Autodesk Inventor part; units mm, degrees
ref_plane "Work Plane1" through (29, 0, 0) normal (0, -1, 0) x (1, 0, 0)
ref_plane "YZ Plane" through (0, 0, 0) normal (1, 0, 0) x (0, 1, 0)
ref_plane "XZ Plane" through (0, 0, 0) normal (0, 1, 0) x (-1, 0, 0)
sketch "Sketch1" plane through (0, 0, 0) normal (0, 0, 1) x (1, 0, 0)
  line L0 (-0.7535, 0) -> (15.875, 0)
  line L1 (15.875, 0) -> (15.875, 1.4224)
  line L2 (15.875, 1.4224) -> (1.5877, 1.4224)
  line L3 (1.5877, 1.4224) -> (0.0001, 1.4224)
  line L4 (0.0001, 1.4224) -> (0, 1.4224)
  line L5 (0, 1.4224) -> (0, 2.3241)
  line L6 (0, 2.3241) -> (-2.8448, 2.3241)
  line L7 (-2.8448, 2.3241) -> (-2.8448, 1.3785)
  line L8 (-2.8448, 1.3785) -> (-1.5494, 1.3785)
  line L9 (-1.5494, 1.3785) -> (-0.7535, 0)
  line L10 (-6.5888, 0) -> (19.619, 0)
  line L11 (0, -0.4648) -> (0, 2.7889)
  line L12 (1.5877, 1.4224) -> (0, 1.4224) construction
  dimension "d1" = 14.2873
  dimension "d2" = 1.5876
  dimension "d3" = 2.8448
  dimension "d4" = 1.2954
  dimension "d5" = 60
  dimension "d6" = 2.8448
  dimension "d7" = 2.8448
  dimension "d8" = 2.757
  dimension "d9" = 4.6482
  dimension "d26" = 15.875
revolve "Body" add sketch "Sketch1" angle 360 about axis through (-0.7535, 0, 0) along (1, 0, 0)
sketch "Sketch2" plane through (-2.8448, 0, 0) normal (-1, 0, 0) x (0, 0, 1)
  circle A0 centre (0, 0) radius 1.3785
  line L0 (0, -3.2537) -> (0, 3.2537)
  line L1 (-3.2537, 0) -> (3.2537, 0)
  line L2 (1.3785, 0) -> (0.6892, -1.1938)
  line L3 (0.6892, -1.1938) -> (-0.6892, -1.1938)
  line L4 (-0.6892, -1.1938) -> (-1.3785, 0)
  line L5 (-1.3785, 0) -> (-0.6892, 1.1938)
  line L6 (-0.6892, 1.1938) -> (0.6892, 1.1938)
  line L7 (0.6892, 1.1938) -> (1.3785, 0)
  point P0 (0, 0)
extrude "Slot" add sketch "Sketch2" against normal up to next contours L7 A0 | A0 L2 | L6 L0 A0 | A0 L0 L3 | L0 L6 A0 | A0 L3 L0 | L4 A0 | A0 L5
fillet "Fillet1" radius 0.2286 1 edges at (-2.8448, -2.3241, 0)
thread "Thread"
chamfer "Chamfer1" distance 0.3785 distance2 0.3785 1 edges at (15.875, -1.4224, 0) measured on face at (15.875, -0.3591, -0.7201)
ref_plane "Work Plane1" through (29, 0, 0) normal (0, -1, 0) x (1, 0, 0)
fillet "Fillet2" radius 0.1016 1 edges at (0.0001, -1.4224, 0)
equation "\"d1\" = GEL"
equation "\"d3\" = KOH"
equation "\"d4\" = INTI"
equation "\"d6\" = GD"
equation "\"d7\" = BDM"
equation "\"d8\" = 1.1547 * SW"
equation "\"d9\" = KOD"
equation "\"d26\" = NLG"
equation "\"d30\" = R"
equation "\"d17\" = RR"
equation "\"d13\" = GEL"
equation "\"d15\" = -0.5 * SPD + 0.5 * GD"
equation "\"d16\" = GUL"
equation "\"GD\" = 2.8448"
equation "\"NLG\" = 15.875"
equation "\"GEL\" = 14.2873"
equation "\"KOD\" = 4.6482"
equation "\"KOH\" = 2.8448"
equation "\"INTI\" = 1.2954"
equation "\"GAL\" = 1.5875"
equation "\"GUL\" = 0.37846"
equation "\"BDM\" = 2.8448"
equation "\"SW\" = 2.3876"
equation "\"RR\" = 0.2286"
equation "\"SPD\" = 2.08788"
equation "\"R\" = 0.1016"
equation "\"PHH\" = 0.127"
equation "\"GD1\" = SPD"
equation "\"THREADDIA\" = 2.8448"
equation "\"FAWI\" = 45deg"
equation "\"KOH1\" = 2.5654"
equation "\"NND\" = 2.8448"
equation "\"TOA\" = 30deg"
equation "\"E0\" = 1.155 * SW"
properties part number "ANSI B18.3 - No. 4 - 40 UNC - 5/8 HS HCS" material "Steel, Mild"
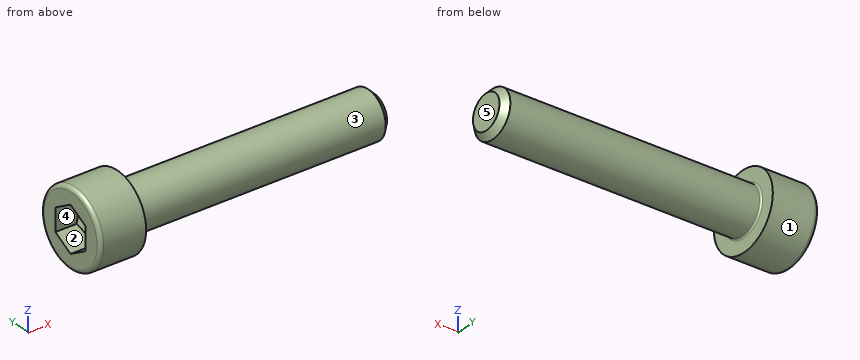
Geometry: final body of the model. Coordinates: model frame, mm. Face numbers are marked on the shaded views. A direction names the side the tool comes from. Give positions to 0.01 mm unless a question says otherwise; leave off trailing zeros. Write each loop counter-clockwise with the first axis right and the second up, starting at its lowest first coordinate (ties: lowest second). Pieces come first, ordered by that corner, then holes. Notation, with made-up numbers: M -30,15 L 19,15 A34 ccw 19,45 Z; hole C 42,70.25 d3. An arc over 180 degrees is marked long. Answer in a Markdown table with one row per item. Add a question column.
(1) Ray query, line 1 (X direction, y = -1.7, z = -0.8); line 2 (Z direction, x = 0.5, y = 0.1); line 3 (X direction, y = -0.15, z = 0.4) (3 decimals). Return the intervals inside material, ascending.
(2) Mould query, pull axis Y, two halves, no side actions, for the marked faces 3, 4 and 5. Classes: +Y half, -Y half, draft (parallel to the pull), parting line (faces both ways), or undercut.
(3) Reachability of the marked faces 1 and 2 from +Z, -Z, +X, -X, +Y, -Y: full face, straight path, thin tool, end or side. Return the list, or none.
(4) Section A-A on x = 4.25. Return loops of the section in (y, z).
Result set:
| question | item | result |
|---|---|---|
| 1 | line 1 | x = -2.84 to 0 |
| 1 | line 2 | z = -1.42 to 1.42 |
| 1 | line 3 | x = -1 to 15.875 |
| 2 | face 3 | parting line |
| 2 | face 4 | undercut |
| 2 | face 5 | draft |
| 3 | face 1 | +X, -X |
| 3 | face 2 | -X |
| 4 | outline | C 0,0 d2.84 |
